Autodesk Inventor part; units mm, degrees
ref_plane "YZ Plane" through (0, 0, 0) normal (1, 0, 0) x (0, 1, 0)
ref_plane "XZ Plane" through (0, 0, 0) normal (0, 1, 0) x (-1, 0, 0)
ref_plane "XY Plane" through (0, 0, 0) normal (0, 0, 1) x (1, 0, 0)
sketch "Sketch1" plane through (0, 0, 0) normal (0, 1, 0) x (-1, 0, 0)
  circle A0 centre (0, 0) radius 10
  dimension "d0" = 20
extrude "Extrusion1" add sketch "Sketch1" along normal blind 14
sketch "Sketch2" plane through (0, 14, 0) normal (0, 1, 0) x (1, 0, 0)
  point P0 (0, 0)
  point P1 (0, 0)
hole "Hole1" at (0, 14, 0) direction (0, -1, 0) diameter 10.376 depth 9 tip angle 118
sketch "Sketch3" plane through (0, 0, 0) normal (0, -1, 0) x (1, 0, 0)
  point P0 (0, 0)
  point P1 (0, 0)
hole "Hole2" at (0, 0, 0) direction (0, 1, 0) diameter 3.9624 end through all
chamfer "Chamfer1" distance 0.6 angle 45 3 edges at (0, 0, 1.9812) (10, 14, 0) (10, 0, 0)
sketch "Sketch4" plane through (0, 0, 0) normal (0, -1, 0) x (1, 0, 0)
  circle A0 centre (0, 0) radius 5.188
  circle A1 centre (0, 0) radius 10
  line L0 (-7.5, 6.6144) -> (7.5, 6.6144)
  line L1 (7.5, 6.6144) -> (7.5, -6.6144)
  line L2 (7.5, -6.6144) -> (-7.5, -6.6144)
  line L3 (-7.5, -6.6144) -> (-7.5, 6.6144)
  circle A2 centre (0, 0) radius 2.5812
  line L4 (-7.5, 6.6144) -> (7.5, -6.6144) construction
  line L5 (7.5, 6.6144) -> (-7.5, -6.6144) construction
  point P0 (-7.5, -6.6144)
  point P1 (-7.5, 6.6144)
  point P2 (7.5, 6.6144)
  dimension "d20" = 15
extrude "Extrusion2" cut sketch "Sketch4" against normal blind 14 contours A1 L1 | L3 A1
properties part number "Port Conversion Nut"
Can you work these out from the model? Positions are in its coordinate system, mm. Give positions to 0.01 mm unless a question says otherwise; leave off trailing zeros. Order: outer loops, then holes, each group sorted by start corner. A loop starts at its lowest first (then second) coordinate and runs counter-clockwise, first axis right, second up. Notation, with made-up numbers: M -5,71 L 34,71 A19 ccw 34,106 Z; hole C -30,-32 d1. An arc over 180 degrees is marked long. One line per item, written item: value.
1) I want a section at A-A, the plane x = 0. List the corners of the cut face in (y, z) for me.
Answer sheet:
outline: M 0,-9.4 L 0.6,-10 L 13.4,-10 L 14,-9.4 L 14,-5.19 L 5,-5.19 L 3.07,-1.98 L 0.6,-1.98 L 0,-2.58 Z; M 0,2.58 L 0.6,1.98 L 3.07,1.98 L 5,5.19 L 14,5.19 L 14,9.4 L 13.4,10 L 0.6,10 L 0,9.4 Z
2) I want a section at B-B, the plane z = 0. List the corners of the cut face in (x, y) for me.
Answer sheet:
outline: M -7.5,0 L -2.58,0 L -1.98,0.6 L -1.98,3.07 L -5.19,5 L -5.19,14 L -7.5,14 Z; M 1.98,0.6 L 2.58,0 L 7.5,0 L 7.5,14 L 5.19,14 L 5.19,5 L 1.98,3.07 Z
3) We'd pull the mould along X, two halves only. Please class faces 1 (the face through (-1.964, 1.854, 0.258)), 2 (the face through (-3.51, 9.44, -3.82)), 3 (the face through (-0.1, 13.8, -9.6)), 4 (the face through (-7.5, 7, 0)): released by +X, released by -X, zero draft, split by the parting line, or undercut.
Answer sheet:
face 1: undercut
face 2: undercut
face 3: split by the parting line
face 4: released by -X
4) I want a section at C-C, the plane y = 6.25. List the corners of the cut face in (x, z) for me.
Answer sheet:
outline: M -7.5,-6.61 A10 ccw 7.5,-6.61 L 7.5,6.61 A10 ccw -7.5,6.61 Z; hole C 0,0 d10.38
5) For P1, Ø2, axis at x = -5, y = 1.5, coming from the -Z side; P2, Ø1, axis at x = -5, y = 1.5, coming from the -Z side; P3, Ø2, axis at x = 4.5, y = 8.5, coming from the +Z side, each with a flat end and sliding along its axis, tell me the tip position at first contact or that it passes through.
Answer sheet:
P1: stops at z = -9.17
P2: stops at z = -8.93
P3: stops at z = 9.37
6) Please list where these lines run through material, in increasing order: line 1 along X through (y, z) = (7.75, 0); line 2 along Z through (x, y) = (0, 12.25); line 3 along Z through (x, y) = (0, 1.1).
Answer sheet:
line 1: x = -7.5 to -5.19, 5.19 to 7.5
line 2: z = -10 to -5.19, 5.19 to 10
line 3: z = -10 to -1.98, 1.98 to 10
